Drawing for the job (mm, zero at the part's lowest x, y, z). Give positions to 0.01 mm unless a question says otherwise; leave off trailing zeros. Loops run counter-clockwise (first coordinate to the right, second up) from the corner with the lowest first, then second, coordinate; pieces in that order, holes last. Notation, with made-up numbers: (60.5, -28) - (112.5, -28) arc R22 ccw to (112.5, 10) - close; hole circle Ø7 at (88.25, 50.25). An arc over 180 degrees is marked (long way). Return JSON: item names as keys, results as strings. Group by question number.
1) Slice it at C-C (z = 0.6). List the corners of the cut face in (x, y).
2) Drill centre lines: probe 1 along X at (y, z) = (10, 3.15); probe 2 along X at (y, z) = (10, 1.15); probe 3 along Y at (x, z) = (25, 0.6). Where is each one in solid material? Low to high. Write a range as from..to.
3) Slice it at A-A (x = 10.5). List the corners of the cut face in (y, z).
4) Mould opens along Y. For the marked faces 1, 2 and 3 say: released by +Y, released by -Y, zero draft, split by the parting line, or undercut.
5) Slice it at B-B (y = 10). List the corners of the cut face in (x, z).
6) Slice it at D-D (y = 12.5). List the corners of the cut face in (x, z).
7) Drop a flat-ended pin along its axis: pin 1 (10 mm diameter, centred on x = 25, y = 10, fed in from +Z). Give the stop position or say it passes through.
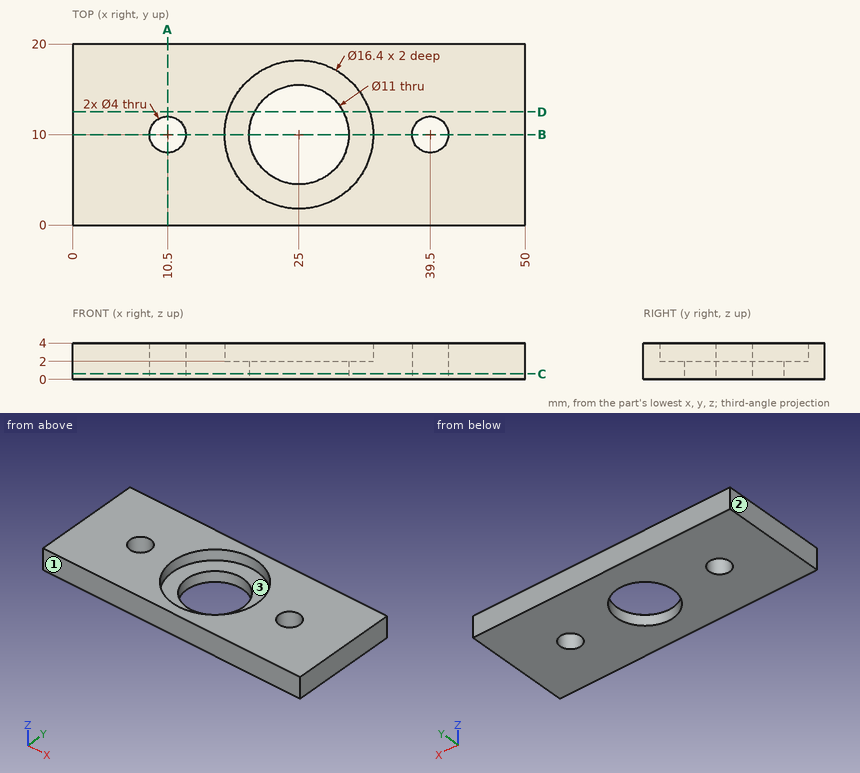
Results:
{
 "1": {"outline": "(0, 0) - (50, 0) - (50, 20) - (0, 20) - close; hole circle Ø4 at (10.5, 10); hole circle Ø11 at (25, 10); hole circle Ø4 at (39.5, 10)"},
 "2": {"probe 1": "0..8.5, 12.5..16.8, 33.2..37.5, 41.5..50", "probe 2": "0..8.5, 12.5..19.5, 30.5..37.5, 41.5..50", "probe 3": "0..4.5, 15.5..20"},
 "3": {"outline": "(0, 0) - (8, 0) - (8, 4) - (0, 4) - close; (12, 0) - (20, 0) - (20, 4) - (12, 4) - close"},
 "4": {"face 1": "released by -Y", "face 2": "zero draft", "face 3": "undercut"},
 "5": {"outline": "(0, 0) - (8.5, 0) - (8.5, 4) - (0, 4) - close; (12.5, 0) - (19.5, 0) - (19.5, 2) - (16.8, 2) - (16.8, 4) - (12.5, 4) - close; (30.5, 0) - (37.5, 0) - (37.5, 4) - (33.2, 4) - (33.2, 2) - (30.5, 2) - close; (41.5, 0) - (50, 0) - (50, 4) - (41.5, 4) - close"},
 "6": {"outline": "(0, 0) - (20.1, 0) - (20.1, 2) - (17.19, 2) - (17.19, 4) - (0, 4) - close; (29.9, 0) - (50, 0) - (50, 4) - (32.81, 4) - (32.81, 2) - (29.9, 2) - close"},
 "7": {"pin 1": "through"}
}
